from build123d import *

# Parameters (mm, degrees)
F0_W     = 50
F0_H     = 50
F0_R     = 3.3
F0_W_2   = 15
F0_H_2   = 20
F1_DEPTH = 8
F0_R_2   = 1.6
F2_DEPTH = 1.75
F3_R     = 2.5


with BuildPart() as f1:
    # F0 (on Top) → F1 (new body)
    with BuildSketch(Plane.XY):
        with Locations((1, -3.352269)):
            Rectangle(F0_W, F0_H)
        with Locations((-19, -23.352269)):
            Circle(F0_R, mode=Mode.SUBTRACT)
        with Locations((21, -23.352269)):
            Circle(F0_R, mode=Mode.SUBTRACT)
        with Locations((-7.5, 8.647731)):
            Rectangle(F0_W_2, F0_H_2, mode=Mode.SUBTRACT)
        with Locations((-19, 16.647731)):
            Circle(F0_R, mode=Mode.SUBTRACT)
        with Locations((21, 16.647731)):
            Circle(F0_R, mode=Mode.SUBTRACT)
    extrude(amount=F1_DEPTH)

    # F0 (on Top) → F2 (join)
    with BuildSketch(Plane.XY):
        with Locations((1, -3.352269)):
            Rectangle(F0_W, F0_H)
        with Locations((-19, -23.352269)):
            Circle(F0_R, mode=Mode.SUBTRACT)
        with Locations((21, -23.352269)):
            Circle(F0_R, mode=Mode.SUBTRACT)
        with Locations((-7.5, 8.647731)):
            Rectangle(F0_W_2, F0_H_2, mode=Mode.SUBTRACT)
        with Locations((-19, 16.647731)):
            Circle(F0_R, mode=Mode.SUBTRACT)
        with Locations((21, 16.647731)):
            Circle(F0_R, mode=Mode.SUBTRACT)
        with Locations((21, 16.647731)):
            Circle(F0_R)
        with Locations((21, 16.647731)):
            Circle(F0_R_2, mode=Mode.SUBTRACT)
        with Locations((-19, 16.647731)):
            Circle(F0_R)
        with Locations((-19, 16.647731)):
            Circle(F0_R_2, mode=Mode.SUBTRACT)
        with Locations((-19, -23.352269)):
            Circle(F0_R)
        with Locations((-19, -23.352269)):
            Circle(F0_R_2, mode=Mode.SUBTRACT)
        with Locations((21, -23.352269)):
            Circle(F0_R)
        with Locations((21, -23.352269)):
            Circle(F0_R_2, mode=Mode.SUBTRACT)
    extrude(amount=F2_DEPTH)

    # F3
    f3_edges = [f1.edges().sort_by_distance(p)[0] for p in [
        (-24, 21.647731, 4),
        (26, 21.647731, 4),
        (26, -28.352269, 4),
        (-24, -28.352269, 4),
    ]]
    fillet(f3_edges, radius=F3_R)


solid = f1.part
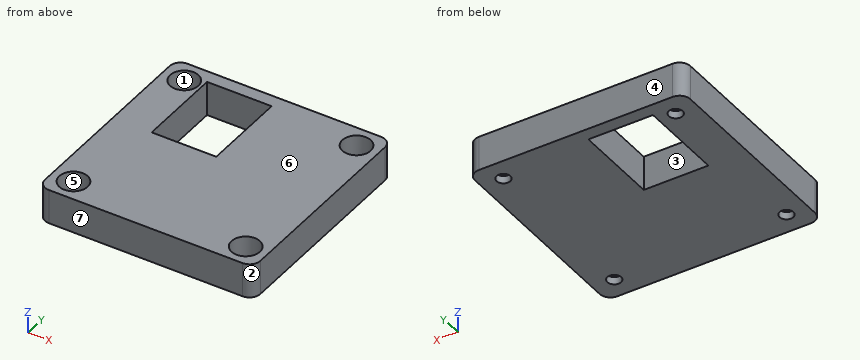
Verification items for the finished model (mm, model axes). Face numbers are marked on the shaded views. A direction names the side the tool comes from. Round coordinates to 2 decimals unless told otherwise and drop trailing zeros. Loops run counter-clockwise (first coordinate to the right, second up) from the corner with the lowest first, then second, coordinate; pieces in that order, holes last. Notation, with made-up numbers: (53, 1.25) - (75, 1.25) arc R11 cw to (75, 18.25) - close; hole circle Ø6 at (-33.5, 81.25). An arc over 180 degrees is marked (long way). Answer in a Markdown table with one row per item. Add a question column.
Q1. Gauge pin test, flat ends, axial feed: pin 1 (5.5 mm diameter, centred on x = 22, y = -23.5, fed in from +Z); pin 2 (2 mm diameter, centred on x = 20, y = 18, fed in from +Z). Record the tip position at first contact, or that the pin passes through.
Q2. Section check A-A on x = 21. Enter the section's corners in (y, z).
Q3. Section check D-D on z = 4.5. Enter the section's corners in (x, y).
Q4. Release check for a two-part mould opening along Y. For the marked faces 4, 5, 6 and 7 record: pulls with the +Y half, pulls with the -Y half, needs draft (parallel to the pull), parting line crosses it, or undercut.
Q5. Tool access check on the marked faces 1, 2 and 3. Record the directions out of +Z, -Z, +X, -X, +Y, -Y that give a thin tool (end or side, any length) a straight path to the whole face; none if there is none.
Q6. Section check C-C on z = 1. Enter the section's corners in (x, y), plus the area to 3 significant figures.
Q7. Section check B-B on x = -7.5. Enter the section's corners in (y, z).
Q8. Material ranges on line 1 (Y direction, x = -19, z = 0.5); line 2 (Y direction, x = 21, z = 5); line 3 (X direction, y = 7.5, z = 2.75), recorded low to high.
Found:
| question | item | result |
|---|---|---|
| 1 | pin 1 | stops at z = 8 |
| 1 | pin 2 | stops at z = 1.75 |
| 2 | outline | (-28.35, 0) - (-24.95, 0) - (-24.95, 1.75) - (-26.65, 1.75) - (-26.65, 8) - (-28.35, 8) - close; (-21.75, 0) - (15.05, 0) - (15.05, 1.75) - (13.35, 1.75) - (13.35, 8) - (-20.05, 8) - (-20.05, 1.75) - (-21.75, 1.75) - close; (18.25, 0) - (21.65, 0) - (21.65, 8) - (19.95, 8) - (19.95, 1.75) - (18.25, 1.75) - close |
| 3 | outline | (-24, -25.85) arc R2.5 ccw to (-21.5, -28.35) - (23.5, -28.35) arc R2.5 ccw to (26, -25.85) - (26, 19.15) arc R2.5 ccw to (23.5, 21.65) - (-21.5, 21.65) arc R2.5 ccw to (-24, 19.15) - close; hole circle Ø6.6 at (-19, -23.35); hole circle Ø6.6 at (-19, 16.65); hole (-15, -1.35) - (0, -1.35) - (0, 18.65) - (-15, 18.65) - close; hole circle Ø6.6 at (21, -23.35); hole circle Ø6.6 at (21, 16.65) |
| 4 | face 4 | pulls with the +Y half |
| 4 | face 5 | undercut |
| 4 | face 6 | needs draft |
| 4 | face 7 | pulls with the -Y half |
| 5 | face 1 | +Z |
| 5 | face 2 | +Z, -Z, +X, -Y |
| 5 | face 3 | +Z, -Z |
| 6 | outline | (-24, -25.85) arc R2.5 ccw to (-21.5, -28.35) - (23.5, -28.35) arc R2.5 ccw to (26, -25.85) - (26, 19.15) arc R2.5 ccw to (23.5, 21.65) - (-21.5, 21.65) arc R2.5 ccw to (-24, 19.15) - close; hole circle Ø3.2 at (-19, -23.35); hole circle Ø3.2 at (-19, 16.65); hole (-15, -1.35) - (0, -1.35) - (0, 18.65) - (-15, 18.65) - close; hole circle Ø3.2 at (21, -23.35); hole circle Ø3.2 at (21, 16.65) |
| 6 | area | 2,160 mm² |
| 7 | outline | (-28.35, 0) - (-1.35, 0) - (-1.35, 8) - (-28.35, 8) - close; (18.65, 0) - (21.65, 0) - (21.65, 8) - (18.65, 8) - close |
| 8 | line 1 | y = -28.35 to -24.95, -21.75 to 15.05, 18.25 to 21.65 |
| 8 | line 2 | y = -28.35 to -26.65, -20.05 to 13.35, 19.95 to 21.65 |
| 8 | line 3 | x = -24 to -15, 0 to 26 |
